Autodesk Inventor part; units mm, degrees
ref_plane "YZ Plane" through (0, 0, 0) normal (1, 0, 0) x (0, 1, 0)
ref_plane "XZ Plane" through (0, 0, 0) normal (0, 1, 0) x (-1, 0, 0)
ref_plane "XY Plane" through (0, 0, 0) normal (0, 0, 1) x (1, 0, 0)
sketch "スケッチ1" plane through (0, 0, 0) normal (0, 0, 1) x (1, 0, 0)
  line L0 (-16, -16) -> (16, -16)
  line L1 (16, -16) -> (16, 16)
  line L2 (16, 16) -> (-16, 16)
  line L3 (-16, 16) -> (-16, -16)
  line L4 (-16, -16) -> (16, 16) construction
  line L5 (16, -16) -> (-16, 16) construction
  line L6 (-14.4, 14.4) -> (14.4, 14.4)
  line L7 (14.4, 14.4) -> (14.4, -14.4)
  line L8 (14.4, -14.4) -> (-14.4, -14.4)
  line L9 (-14.4, -14.4) -> (-14.4, 14.4)
  point P0 (0, 0)
  dimension "d0" = 32
  dimension "d1" = 32
  dimension "d2" = 1.6
extrude "押し出し1" add sketch "スケッチ1" along normal blind 127.5
sketch "スケッチ2" plane through (16, -16, 127.5) normal (1, 0, 0) x (0, 0, -1)
  line L0 (0, 0) -> (0, 32)
  point P0 (127.5, 16)
  point P1 (111.5, 16)
  dimension "d8" = 111.5
hole "穴1" at (16, 0, 16) direction (-1, 0, 0) diameter 10.5 end through all
properties part number "PipeB"
The listing builds one solid part. Answer for the finished solid, in the listing's coordinates (mm). A direction names the side the tool comes from. Give positions to 0.01 mm unless a question says otherwise; leave off trailing zeros. Loops run counter-clockwise (first coordinate to the right, second up) from the corner with the lowest first, then second, coordinate; pieces in that order, holes last.
Item 1: A tool of negligible diameter and unlimited length cuts with its end or side. For faces 4 (the flat face through (-16, 0, 63)), 5 (the flat face through (0, 14.4, 63)), from which of +Z, -Z, +X, -X, +Y, -Y can it reach the whole face along a straight path? Write none if from no direction.
Derived:
face 4: +Z, -Z, -X, +Y, -Y
face 5: +Z, -Z
Item 2: A cutting plane is placed at C-C (x = -6). Give the vertices of the cut face in (y, z), then the cut area to 3 significant figures.
Derived:
outline: (-16, 0) - (-14.4, 0) - (-14.4, 127.5) - (-16, 127.5) - close; (14.4, 0) - (16, 0) - (16, 127.5) - (14.4, 127.5) - close
area: 408 mm2
Item 3: A cutting plane is placed at A-A (y = 0). Give the vertices of the cut face in (x, z).
Derived:
outline: (-16, 0) - (-14.4, 0) - (-14.4, 10.75) - (-16, 10.75) - close; (-16, 21.25) - (-14.4, 21.25) - (-14.4, 127.5) - (-16, 127.5) - close; (14.4, 0) - (16, 0) - (16, 10.75) - (14.4, 10.75) - close; (14.4, 21.25) - (16, 21.25) - (16, 127.5) - (14.4, 127.5) - close
Item 4: This flat-tipped pin is pushed along its axis until it touches: pin 1 Ø6.5 at (y, z) = (0, 16) entering from -X. Where does it stop, or does it pass through?
Derived:
pin 1: passes through
Item 5: A cutting plane is placed at B-B (z = 16). Give the vertices of the cut face in (x, y), then the cut area to 3 significant figures.
Derived:
outline: (-16, -16) - (16, -16) - (16, -5.25) - (14.4, -5.25) - (14.4, -14.4) - (-14.4, -14.4) - (-14.4, -5.25) - (-16, -5.25) - close; (-16, 5.25) - (-14.4, 5.25) - (-14.4, 14.4) - (14.4, 14.4) - (14.4, 5.25) - (16, 5.25) - (16, 16) - (-16, 16) - close
area: 161 mm2
Item 6: Determine the mould class of faces 1 (the cylindrical face through (15.189, -0.231, 21.245)), 2 (the flat face through (-1, -15, 0)), 3 (the flat face through (-14.4, 0, 63)) for opening direction Z: +Z half, -Z half, draft (parallel to the pull), parting line (faces both ways), or undercut.
Derived:
face 1: undercut
face 2: -Z half
face 3: draft
Item 7: Find the intervals of material crossed by line 1 along Y through (x, z) = (-15, 16); line 2 along X through (y, z) = (14, 11), in increasing order.
Derived:
line 1: y = -16 to -5.25, 5.25 to 16
line 2: x = -16 to -14.4, 14.4 to 16
